For this review, take the finished solid that the model builds, in its own axes (mm). A direction names the side the tool comes from. Round coordinates to 2 decimals unless told otherwise and drop trailing zeros. Loops run counter-clockwise (first coordinate to the right, second up) from the corner with the lowest first, then second, coordinate; pieces in that order, holes last. Notation, with made-up numbers: (87.25, 36.5) -> (145.25, 36.5) arc R21 ccw to (145.25, 52.5) -> close; hole circle Ø9 at (-20, -34.5). An arc over 180 degrees is marked (long way). Write each question's results on one line, items separated by ' | '.
Autodesk Inventor part; units mm, degrees
ref_plane "РабПлоскость1" through (0, 250, 0) normal (0, 1, 0) x (1, 0, 0)
ref_plane "YZ Plane" through (0, 0, 0) normal (1, 0, 0) x (0, 1, 0)
ref_plane "XZ Plane" through (0, 0, 0) normal (0, 1, 0) x (-1, 0, 0)
sketch "Эскиз1" plane through (0, 0, 0) normal (0, 1, 0) x (-1, 0, 0)
  line L0 (20.5571, -2.4) -> (-16.8429, -2.4)
  line L1 (-21.6429, -7.2) -> (-21.6429, -7.2)
  line L2 (-16.8429, -12) -> (20.5571, -12)
  line L3 (25.3571, -7.2) -> (25.3571, -7.2)
  arc A0 (25.3571, -7.2) -> (20.5571, -2.4) centre (20.5571, -7.2) ccw
  arc A1 (20.5571, -12) -> (25.3571, -7.2) centre (20.5571, -7.2) ccw
  arc A2 (-16.8429, -2.4) -> (-21.6429, -7.2) centre (-16.8429, -7.2) ccw
  arc A3 (-21.6429, -7.2) -> (-16.8429, -12) centre (-16.8429, -7.2) ccw
  line L4 (19.0571, -3.4) -> (-15.3429, -3.4)
  line L5 (-19.1429, -7.2) -> (-19.1429, -7.2)
  line L6 (-15.3429, -11) -> (19.0571, -11)
  line L7 (22.8571, -7.2) -> (22.8571, -7.2)
  arc A4 (22.8571, -7.2) -> (19.0571, -3.4) centre (19.0571, -7.2) ccw
  arc A5 (19.0571, -11) -> (22.8571, -7.2) centre (19.0571, -7.2) ccw
  arc A6 (-19.1429, -7.2) -> (-15.3429, -11) centre (-15.3429, -7.2) ccw
  arc A7 (-15.3429, -3.4) -> (-19.1429, -7.2) centre (-15.3429, -7.2) ccw
  point P0 (0, 0)
  point P1 (25.3571, -2.4)
  point P2 (-21.6429, -2.4)
  dimension "d0" = 47
  dimension "d1" = 9.6
  dimension "d2" = 4.8
  dimension "d3" = 1
  dimension "d4" = 1
  dimension "d5" = 2.5
  dimension "d6" = 2.5
  dimension "d7" = 3.8
extrude "Выдавливание1" add sketch "Эскиз1" along normal blind 240
ref_plane "РабПлоскость1" through (0, 250, 0) normal (0, 1, 0) x (1, 0, 0)
fillet "Сопряжение1" radius 0.5 8 edges at (18.0299, 0, -9.887) (-1.8571, 0, -11) (-21.7441, 0, -9.887) (-1.8571, 0, -3.4) (-23.9513, 0, -3.8059) (-1.8571, 0, -12) (20.237, 0, -3.8059) (-1.8571, 0, -2.4)
fillet "Сопряжение2" radius 0.5 8 edges at (20.237, 240, -10.5941) (-1.8571, 240, -12) (-23.9513, 240, -3.8059) (-1.8571, 240, -2.4) (-21.7441, 240, -9.887) (-1.8571, 240, -11) (18.0299, 240, -9.887) (-1.8571, 240, -3.4)
sketch3d "3D эскиз1"
ref_plane "РабПлоскость9" through (-10.4571, 0, -2.9) normal (0, -1, 0) x (1, 0, 0)
ref_plane "РабПлоскость10" through (-24.8571, 240, -7.2) normal (0, 1, 0) x (1, 0, 0)
properties part number "isolator_A"
1. Draft analysis for pull direction Z (two halves, no side actions). For faces 1 (the face through (-2, 118, -11)), 2 (the face through (-2, 118, -2.4)), 3 (the face through (-2, 118, -12)), state which applies: released by +Z, released by -Z, zero draft, split by the parting line, or undercut.
Values found:
face 1: undercut | face 2: released by +Z | face 3: released by -Z
2. To check wall thickness, follow probe 1 along Z at (x, y) = (-2, 202); probe 2 along X at (y, z) = (78, -7); probe 3 along X at (y, z) = (129.5, -5.25). State the ranges of each line that lie inside material, in increasing order.
Values found:
probe 1: z = -12 to -11, -3.4 to -2.4 | probe 2: x = -25.35 to -22.85, 19.14 to 21.64 | probe 3: x = -24.94 to -22.32, 18.6 to 21.23
3. Consider section B-B (y = 108). State the section outline as (x, z) points, plus the area to 3 significant figures.
Values found:
outline: (-20.56, -12) -> (16.84, -12) arc R4.8 ccw to (16.84, -2.4) -> (-20.56, -2.4) arc R4.8 ccw to start; hole (-19.06, -11) -> (15.34, -11) arc R3.8 ccw to (15.34, -3.4) -> (-19.06, -3.4) arc R3.8 ccw to start | area: 125 mm2
4. Tool access review of faces 4 (the face through (-22.2, 0, -4)), 5 (the face through (19.142, 118.327, -7.284)): name each direction out of +Z, -Z, +X, -X, +Y, -Y from which nothing blocks a thin tool from reaching the whole face with its end or side.
Values found:
face 4: +Z, -Z, +X, -X, -Y | face 5: +Y, -Y
5. Consider section C-C (z = -7.2). State the section outline as (x, y) points.
Values found:
outline: (-25.36, 0.5) arc R0.5 ccw to (-24.86, 0) -> (-23.36, 0) arc R0.5 ccw to (-22.86, 0.5) -> (-22.86, 239.5) arc R0.5 ccw to (-23.36, 240) -> (-24.86, 240) arc R0.5 ccw to (-25.36, 239.5) -> close; (19.14, 0.5) arc R0.5 ccw to (19.64, 0) -> (21.14, 0) arc R0.5 ccw to (21.64, 0.5) -> (21.64, 239.5) arc R0.5 ccw to (21.14, 240) -> (19.64, 240) arc R0.5 ccw to (19.14, 239.5) -> close
6. For pin 1 (1 mm diameter, centred on x = -15, z = -5.5, fed in from -Y); pin 2 (1.5 mm diameter, centred on y = 166.5, z = -9.5, fed in from -X); pin 3 (3 mm diameter, centred on y = 26.5, z = -4, fed in from -X), all flat-tipped, find the tip position at first contact; note any pin that passes through.
Values found:
pin 1: passes through | pin 2: stops at x = -25.1 | pin 3: stops at x = -25.05
